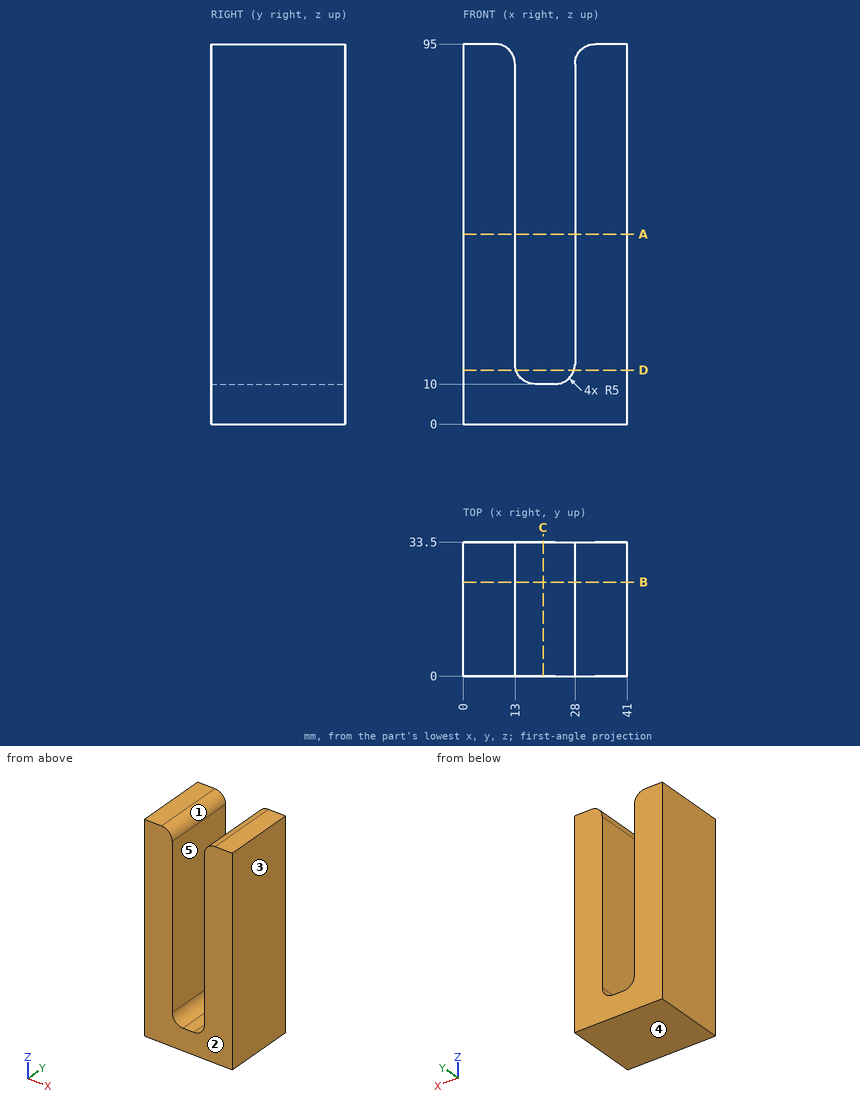
Input: dimensioned drawing with shaded views. Units: mm. Origin: part minimum x, y, z. A direction names the side the tool comes from. Coordinates: 2 decimals unless noted, no trailing zeros. Loops run counter-clockwise (first coordinate to the right, second up) from the corner with the lowest first, then second, coordinate; pieces in that order, holes last. Notation, with made-up numbers: M 6,-28.75 L 16,-28.75 A17 ccw 16,-10.75 Z; hole C -30,62.25 d10. An arc over 180 degrees is marked long. Use a Markdown table: item, result. Add a question column.
Q1. Draft query along X for the marked faces 1, 2 and 3. Return one class per face: pulls with the +X half, pulls with the -X half, needs draft (parallel to the pull), parting line crosses it, or undercut.
Q2. Section query A-A, the plane z = 47.5. Return loops of the section in (x, y).
Q3. First-contact query: pin 1 (1 mm diameter, centred on y = 10, z = 75.5, fed in from -X); pin 2 (5 mm diameter, centred on x = 21, y = 26.5, fed in from +Z). Flat tips, straight axial feed; report the tip coordinate or a pass-through.
Q4. Section query D-D, the plane z = 13.5. Return loops of the section in (x, y), and give its area (3 significant figures).
Q5. Section query B-B, the plane y = 23.5. Return loops of the section in (x, z).
Q6. Access query for the marked faces 4 and 5. Directions: +Z, -Z, +X, -X, +Y, -Y. A direction counts if a zero-diameter tool reaches every point of the face in a straight line with its end or side. Return the directions, or none.
Q7. Section query C-C, the plane x = 20. Return loops of the section in (y, z).
Q8. Material intervals for L1, parallel to X at y = 26, z = 54; L2, parallel to X at y = 20, z = 10.5; L3, parallel to Z at x = 20, y = 11, sorted ascending.
Result:
| question | item | result |
|---|---|---|
| 1 | face 1 | undercut |
| 1 | face 2 | needs draft |
| 1 | face 3 | pulls with the +X half |
| 2 | outline | M 0,0 L 13,0 L 13,33.5 L 0,33.5 Z; M 28,0 L 41,0 L 41,33.5 L 28,33.5 Z |
| 3 | pin 1 | stops at x = 0 |
| 3 | pin 2 | stops at z = 10.03 |
| 4 | outline | M 0,0 L 13.23,0 L 13.23,33.5 L 0,33.5 Z; M 27.77,0 L 41,0 L 41,33.5 L 27.77,33.5 Z |
| 4 | area | 886 mm2 |
| 5 | outline | M 0,0 L 41,0 L 41,95 L 33,95 A5 ccw 28,90 L 28,15 A5 cw 23,10 L 18,10 A5 cw 13,15 L 13,90 A5 ccw 8,95 L 0,95 Z |
| 6 | face 4 | -Z, +X, -X, +Y, -Y |
| 6 | face 5 | +Z, +Y, -Y |
| 7 | outline | M 0,0 L 33.5,0 L 33.5,10 L 0,10 Z |
| 8 | L1 | x = 0 to 13, 28 to 41 |
| 8 | L2 | x = 0 to 15.82, 25.18 to 41 |
| 8 | L3 | z = 0 to 10 |
